from build123d import *

# Parameters (mm, degrees)
SKETCH_1_W          = 23.1
SKETCH_1_H          = 18.6
EXTRUDE_1_DEPTH     = 1.5
SKETCH_2_R          = 0.75
SKETCH_2_R_2        = 1
SKETCH_2_R_3        = 0.35
CUT_EXTRUDE_1_DEPTH = 15.904445646
SKETCH_3_W          = 3
SKETCH_3_H          = 3
SKETCH_3_R          = 0.6
EXTRUDE_2_DEPTH     = 1.5


with BuildPart() as part:
    # 草图1 → 凸台-拉伸1 (new body)
    with BuildSketch(Plane.XY):
        Rectangle(SKETCH_1_W, SKETCH_1_H)
    extrude(amount=EXTRUDE_1_DEPTH)

    # 草图2 → 切除-拉伸1 (cut, through all)
    with BuildSketch(Plane(origin=(0, 0, 0), x_dir=(-1, 0, 0), z_dir=(0, 0, -1))):
        with Locations((-10.6, 2.5)):
            Circle(SKETCH_2_R)
        with Locations((-10.6, 0)):
            Circle(SKETCH_2_R)
        with Locations((-10.6, -2.5)):
            Circle(SKETCH_2_R)
        with Locations((-7.55, -6.3)):
            Circle(SKETCH_2_R_2)
        with Locations((3.15, -6.3)):
            Circle(SKETCH_2_R_2)
        with Locations((-4.7, -8.4)):
            Circle(SKETCH_2_R)
        with Locations((-2.2, -8.4)):
            Circle(SKETCH_2_R)
        with Locations((0.3, -8.4)):
            Circle(SKETCH_2_R)
        with Locations((-7.55, 6.3)):
            Circle(SKETCH_2_R_2)
        with Locations((3.15, 6.3)):
            Circle(SKETCH_2_R_2)
        with Locations((5.6, 3.2)):
            Circle(SKETCH_2_R)
        with Locations((9.8, 3.2)):
            Circle(SKETCH_2_R)
        with Locations((5.6, -3.2)):
            Circle(SKETCH_2_R)
        with Locations((9.8, -3.2)):
            Circle(SKETCH_2_R)
        with Locations((5.7, -7.9)):
            Circle(SKETCH_2_R_3)
        with Locations((-10.1, -7.9)):
            Circle(SKETCH_2_R_3)
        with Locations((-10.1, 7.9)):
            Circle(SKETCH_2_R_3)
    extrude(amount=-CUT_EXTRUDE_1_DEPTH, mode=Mode.SUBTRACT)

    # 草图3 → 凸台-拉伸2 (add)
    # profile 1 of 4: a face of its own
    with BuildSketch(Plane(origin=(0, 0, 0), x_dir=(-1, 0, 0), z_dir=(0, 0, -1))):
        with Locations((-13.05, 7.8)):
            Rectangle(SKETCH_3_W, SKETCH_3_H)
        with Locations((-13.05, 7.8)):
            Circle(SKETCH_3_R, mode=Mode.SUBTRACT)
    # profile 2 of 4: a face of its own
    with BuildSketch(Plane(origin=(0, 0, 0), x_dir=(-1, 0, 0), z_dir=(0, 0, -1))):
        with Locations((-13.05, -7.8)):
            Rectangle(SKETCH_3_W, SKETCH_3_H)
        with Locations((-13.05, -7.8)):
            Circle(SKETCH_3_R, mode=Mode.SUBTRACT)
    # profile 3 of 4: a face of its own
    with BuildSketch(Plane(origin=(0, 0, 0), x_dir=(-1, 0, 0), z_dir=(0, 0, -1))):
        with Locations((13.05, 7.8)):
            Rectangle(SKETCH_3_W, SKETCH_3_H)
        with Locations((13.05, 7.8)):
            Circle(SKETCH_3_R, mode=Mode.SUBTRACT)
    # profile 4 of 4: a face of its own
    with BuildSketch(Plane(origin=(0, 0, 0), x_dir=(-1, 0, 0), z_dir=(0, 0, -1))):
        with Locations((13.05, -7.8)):
            Rectangle(SKETCH_3_W, SKETCH_3_H)
        with Locations((13.05, -7.8)):
            Circle(SKETCH_3_R, mode=Mode.SUBTRACT)
    extrude(amount=-EXTRUDE_2_DEPTH)


solid = part.part
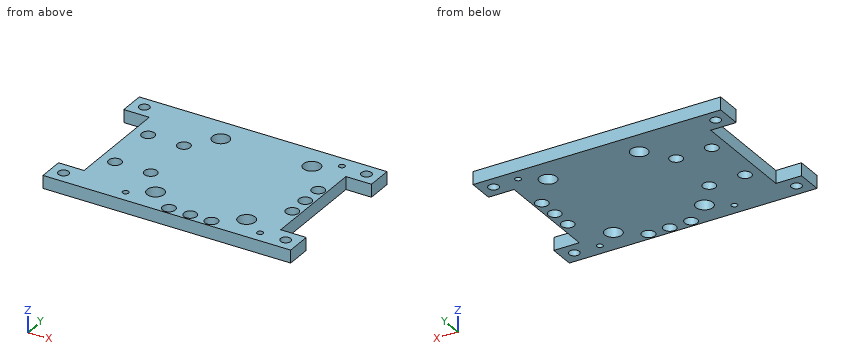
The listing builds one solid part. Answer for the finished solid, in the listing's coordinates (mm). Coordinates: 2 decimals unless noted, no trailing zeros. Loops run counter-clockwise (first coordinate to the right, second up) from the corner with the lowest first, then second, coordinate; pieces in that order, holes last.
1) Find section B-B on x = -13.05. Write down the section's boundary in (y, z), then the cut area to 3 significant figures.
2) Find section D-D on x = -9.8. Write down the section's boundary in (y, z).
3) Find section C-C on z = 0.3. Give the number of separate pieces and of enclosed holes in the cut face, then the cut area to 3 significant figures.
4) Find section A-A on x = 2.2. Write down the section's boundary in (y, z).
5) Find the intervals of material crossed by L1, parallel to Y at x = 7.55, z = 1.15; L2, parallel to Y at x = 10.6, z = 0.6; L3, parallel to X at y = 8, z = 0.55, in increasing order.
Values:
1. outline: (-9.3, 0) - (-8.4, 0) - (-8.4, 1.5) - (-9.3, 1.5) - close; (-7.2, 0) - (-6.3, 0) - (-6.3, 1.5) - (-7.2, 1.5) - close; (6.3, 0) - (7.2, 0) - (7.2, 1.5) - (6.3, 1.5) - close; (8.4, 0) - (9.3, 0) - (9.3, 1.5) - (8.4, 1.5) - close
1. area: 5.40 mm2
2. outline: (-9.3, 0) - (-3.95, 0) - (-3.95, 1.5) - (-9.3, 1.5) - close; (-2.45, 0) - (2.45, 0) - (2.45, 1.5) - (-2.45, 1.5) - close; (3.95, 0) - (9.3, 0) - (9.3, 1.5) - (3.95, 1.5) - close
3. separate pieces: 1
3. enclosed holes: 21
3. area: 430 mm2
4. outline: (-9.3, 0) - (-9.15, 0) - (-9.15, 1.5) - (-9.3, 1.5) - close; (-7.65, 0) - (9.3, 0) - (9.3, 1.5) - (-7.65, 1.5) - close
5. L1: y = -9.3 to -7.3, -5.3 to 5.3, 7.3 to 9.3
5. L2: y = -9.3 to -3.25, -1.75 to -0.75, 0.75 to 1.75, 3.25 to 9.3
5. L3: x = -14.55 to -13.62, -12.48 to 9.76, 10.44 to 12.48, 13.62 to 14.55
